For this review, take the finished solid that the model builds, in its own axes (mm). Face numbers are marked on the shaded views. A direction names the side the tool comes from. Round coordinates to 2 decimals unless told otherwise and drop trailing zeros. Order: outer loops, then holes, each group sorted by start corner. A loop starts at its lowest first (then second) coordinate and runs counter-clockwise, first axis right, second up. Notation, with made-up numbers: (45, 47.25) - (71, 47.25) arc R24 cw to (71, 63.25) - close; hole circle Ø2 at (10.25, 44). An arc over 180 degrees is marked (long way). One line per question, with ' | ' between items.
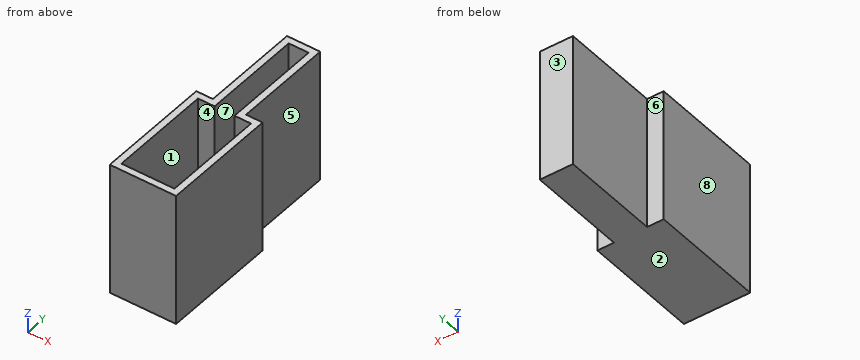
```python
from build123d import *

# Parameters (mm, degrees)
F1_DEPTH = 50.8
F2_T     = -2.54


with BuildPart() as f1:
    # F0 (on Top) → F1 (new body)
    with BuildSketch(Plane.XY):
        Polygon((0, 44.45), (0, 0), (25.4, 0), (25.4, 44.45), (19.05, 44.45), (19.05, 82.55), (6.35, 82.55), (6.35, 44.45), align=None)
    extrude(amount=F1_DEPTH)

    # F2
    f2_openings = [f1.faces().sort_by_distance(p)[0] for p in [
        (12.7, 34.6075, 50.8),
    ]]
    offset(amount=F2_T, openings=f2_openings, kind=Kind.INTERSECTION)


solid = f1.part
```
(1) We need section A-A on z = 30. State the section outline as (x, y) points.
Output values:
outline: (0, 0) - (25.4, 0) - (25.4, 44.45) - (19.05, 44.45) - (19.05, 82.55) - (6.35, 82.55) - (6.35, 44.45) - (0, 44.45) - close; hole (2.54, 2.54) - (22.86, 2.54) - (22.86, 41.91) - (16.51, 41.91) - (16.51, 80.01) - (8.89, 80.01) - (8.89, 41.91) - (2.54, 41.91) - close
(2) For the marked faces 5, 6, 7 and 8, list the 3-axis set-ups (+Z, -Z, +X, -X, +Y, -Y) from which the entire face can be reached by the end or side of a thin tool; tool diameter is ignored.
Output values:
face 5: +Z, -Z, +X, +Y | face 6: +Z, -Z, -X, +Y | face 7: +Z | face 8: +Z, -Z, -X, +Y, -Y
(3) Mouldability with a two-part tool opening along Y and no side actions: class the marked faces 1, 2, 3 and 4 as released by +Y, released by -Y, zero draft, split by the parting line, or undercut.
Output values:
face 1: undercut | face 2: zero draft | face 3: released by +Y | face 4: undercut
(4) We need section B-B on y = 65.5. State the section outline as (x, z) points.
Output values:
outline: (6.35, 0) - (19.05, 0) - (19.05, 50.8) - (16.51, 50.8) - (16.51, 2.54) - (8.89, 2.54) - (8.89, 50.8) - (6.35, 50.8) - close
(5) We need section C-C on x = 11.5. State the section outline as (y, z) points.
Output values:
outline: (0, 0) - (82.55, 0) - (82.55, 50.8) - (80.01, 50.8) - (80.01, 2.54) - (2.54, 2.54) - (2.54, 50.8) - (0, 50.8) - close
(6) For probe 1 along X at (y, z) = (25, 28); probe 2 along Y at (x, z) = (7.5, 8); probe 3 along X at (y, z) = (62, 10), list the stretches that pass through material, from the lowest coordinate up. Write a range as [from, to].
Output values:
probe 1: [0, 2.54], [22.86, 25.4] | probe 2: [0, 2.54], [41.91, 82.55] | probe 3: [6.35, 8.89], [16.51, 19.05]
(7) Insertion check: pin 1 (11.5 mm diameter, centred on y = 68, z = 20.5, fed in from +X); pin 2 (4 mm diameter, centred on y = 57, z = 11.5, fed in from -X); pin 3 (3 mm diameter, centred on x = 3, z = 33.5, fed in from +Y); pin 4 (2 mm diameter, centred on x = 5, y = 47.5, fed in from +Z). Each pin has a flat end and moves straight along its axis. Give the tip position at first contact, or say it passes through.
Output values:
pin 1: x = 19.05 | pin 2: x = 6.35 | pin 3: y = 44.45 | pin 4: through
